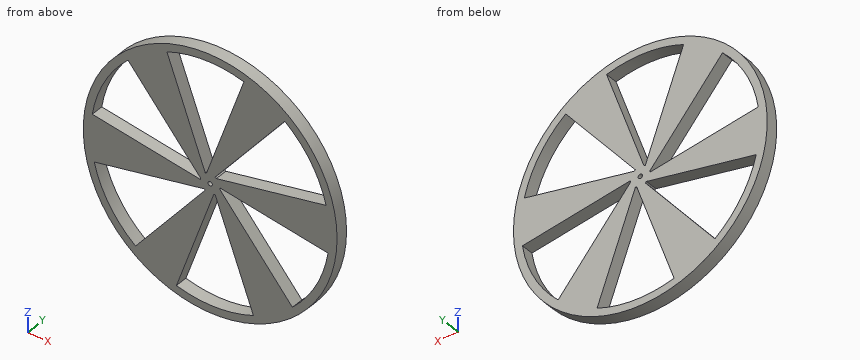
```python
from build123d import *

# Parameters (mm, degrees)
SKETCH1_R           = 50
SKETCH1_R_2         = 47
SKETCH1_R_3         = 3.85
SKETCH1_R_4         = 0.85
BOSS_EXTRUDE1_DEPTH = 5


with BuildPart() as part:
    # Sketch1 → Boss-Extrude1 (new body)
    with BuildSketch(Plane(origin=(0, 0, 0), x_dir=(1, 0, 0), z_dir=(0, 1, 0))):
        Circle(SKETCH1_R)
        Circle(SKETCH1_R_2, mode=Mode.SUBTRACT)
        Circle(SKETCH1_R_3)
        Circle(SKETCH1_R_4, mode=Mode.SUBTRACT)
        with BuildLine():
            ThreePointArc((1.925, -3.334197805), (0.295727162, -3.838625463), (-1.39158336, -3.589706917))
            Line((-1.39158336, -3.589706917), (13.299862292, -45.078971406))
            ThreePointArc((13.299862292, -45.078971406), (21.761273299, -41.658696384), (29.402141879, -36.667615861))
            Line((29.402141879, -36.667615861), (1.925, -3.334197805))
        make_face()
        with BuildLine():
            Line((46.456157771, 7.129193862), (3.85, 0))
            ThreePointArc((3.85, 0), (3.472210748, -1.663205496), (2.412985702, -3))
            Line((2.412985702, -3), (45.68946556, -11.021467091))
            ThreePointArc((45.68946556, -11.021467091), (46.671216404, -5.549554878), (47, 0))
            ThreePointArc((47, 0), (46.86384222, 3.574953479), (46.456157771, 7.129193862))
        make_face()
        with BuildLine():
            Line((17.054015892, 43.796809723), (1.925, 3.334197805))
            ThreePointArc((1.925, 3.334197805), (3.176483585, 2.175419967), (3.804569063, 0.589706917))
            Line((3.804569063, 0.589706917), (32.389603268, 34.057504315))
            ThreePointArc((32.389603268, 34.057504315), (25.196852708, 39.675163687), (17.054015892, 43.796809723))
        make_face()
        with BuildLine():
            Line((-29.402141879, 36.667615861), (-1.925, 3.334197805))
            ThreePointArc((-1.925, 3.334197805), (-0.295727162, 3.838625463), (1.39158336, 3.589706917))
            Line((1.39158336, 3.589706917), (-13.299862292, 45.078971406))
            ThreePointArc((-13.299862292, 45.078971406), (-21.761273299, 41.658696384), (-29.402141879, 36.667615861))
        make_face()
        with BuildLine():
            ThreePointArc((-3.85, 0), (-3.472210748, 1.663205496), (-2.412985702, 3))
            Line((-2.412985702, 3), (-45.68946556, 11.021467091))
            ThreePointArc((-45.68946556, 11.021467091), (-46.958126006, 1.983532697), (-46.456157771, -7.129193862))
            Line((-46.456157771, -7.129193862), (-3.85, 0))
        make_face()
        with BuildLine():
            ThreePointArc((-1.925, -3.334197805), (-3.176483585, -2.175419967), (-3.804569063, -0.589706917))
            Line((-3.804569063, -0.589706917), (-32.389603268, -34.057504315))
            ThreePointArc((-32.389603268, -34.057504315), (-25.196852708, -39.675163687), (-17.054015892, -43.796809723))
            Line((-17.054015892, -43.796809723), (-1.925, -3.334197805))
        make_face()
    extrude(amount=BOSS_EXTRUDE1_DEPTH)


solid = part.part
```
CAD build for the part. Positions are in the model's coordinates, mm. Coordinates: 2 decimals unless noted, no trailing zeros. Order: outer loops, then holes, each group sorted by start corner. A loop starts at its lowest first (then second) coordinate and runs counter-clockwise, first axis right, second up.
(1) Pin check, flat tips, straight feed: pin 1 Ø2 at (x, z) = (-9.5, 28) entering from -Y; pin 2 Ø1.5 at (y, z) = (4, -20) entering from -X. Stop position of each tip, or through.
Solution:
pin 1: passes through
pin 2: stops at x = -46.15
(2) Saw through at B-B, the plane x = 21.5. Write the cut outline in (y, z), and give its area (3 significant figures).
Solution:
outline: (0, -45.14) - (5, -45.14) - (5, -21.31) - (0, -21.31) - close; (0, -2.95) - (5, -2.95) - (5, 6.54) - (0, 6.54) - close; (0, 27.08) - (5, 27.08) - (5, 45.14) - (0, 45.14) - close
area: 257 mm2
(3) Saw through at D-D, the plane x = -10.5. Write the cut outline in (y, z).
Solution:
outline: (0, -48.89) - (5, -48.89) - (5, -45.81) - (0, -45.81) - close; (0, -37.17) - (5, -37.17) - (5, -13.74) - (0, -13.74) - close; (0, -4.5) - (5, -4.5) - (5, 1.11) - (0, 1.11) - close; (0, 8.43) - (5, 8.43) - (5, 26.27) - (0, 26.27) - close; (0, 45.81) - (5, 45.81) - (5, 48.89) - (0, 48.89) - close
(4) Drill centre lines: L1, parallel to X at y = 3.65, z = -27; L2, parallel to Z at x = -36, y = 1.95; L3, parallel to X at y = 4.7, z = -18.5. Where is each one in solid material? Low to high.
Solution:
L1: x = -42.08 to -38.47, -21.43 to -6.9, 10.77 to 26.36, 38.47 to 42.08
L2: z = -34.7 to -30.22, -9.23 to 5.38, 30.22 to 34.7
L3: x = -46.45 to -43.21, -14.43 to -3.89, 7.6 to 19.1, 43.21 to 46.45
(5) Saw through at C-C, the plane z = -26. Write the cut outline in (x, y).
Solution:
outline: (-42.71, 0) - (-39.15, 0) - (-39.15, 5) - (-42.71, 5) - close; (-20.61, 0) - (-6.54, 0) - (-6.54, 5) - (-20.61, 5) - close; (10.4, 0) - (25.51, 0) - (25.51, 5) - (10.4, 5) - close; (39.15, 0) - (42.71, 0) - (42.71, 5) - (39.15, 5) - close
(6) Saw through at A-A, the plane y = 3.45. Count the separate pieces of the cut face and the enclosed holes in it, and give its area (3 significant figures).
Solution:
separate pieces: 1
enclosed holes: 7
area: 3,750 mm2
